Input: dimensioned drawing with shaded views. Units: mm. Origin: part minimum x, y, z. A direction names the side the tool comes from. Give positions to 0.01 mm unless a question says otherwise; leave off trailing zeros. Write each loop counter-clockwise with the first axis right and the second up, starting at its lowest first coordinate (ties: lowest second). Pieces come first, ordered by that corner, then holes. Notation, with made-up numbers: M 25.25,-30 L 34.25,-30 A8 cw 34.25,-16 Z; hole C -34.5,22 d9. An arc over 180 degrees is marked long. Use CSV: the item, a comma, the result in double quotes. Start each with the question number.
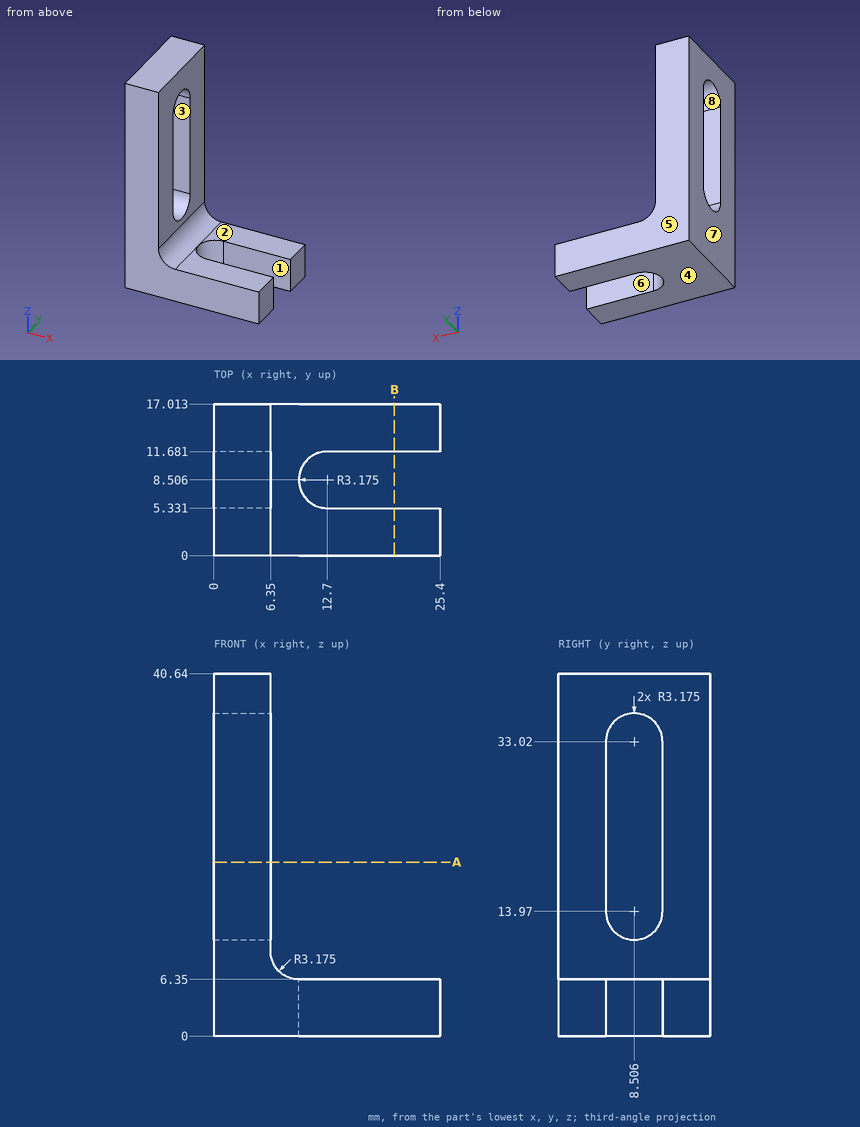
Q1. Section B-B, the plane x = 20.25. Return the cut outline in (y, z).
Q2. Set-up query: the marked faces 1, 2, 3 and 4. Return all of +Z, -Z, +X, -X, +Y, -Y with unobstructed straight access to the full face (end or side cutting, diameter ignored); none if empty.
Q3. Pull-direction query (Y, two-part tool) for the marked faces 5, 6, 7 and 8; classes: released by +Y, released by -Y, zero draft, split by the parting line, or undercut.
Q4. Material intervals for L1, parallel to X at y = 2, z = 32.5; L2, parallel to Z at x = 5.25, y = 7 (1 decimal), sorted ascending. Write a range as [from, to].
Q5. First-contact query: pin 1 Ø5 at (y, z) = (12.5, 36.5) entering from +X; pin 2 Ø4 at (y, z) = (4, 9) entering from +X; pin 3 Ø2.5 at (x, y) = (14.5, 14) entering from +Z. Flat tips, straight axial feed; report the tip coordinate or a pass-through.
Q6. Section A-A, the plane z = 19.5. Return the cut outline in (x, y).
Check result:
1,outline,"M 0,0 L 5.33,0 L 5.33,6.35 L 0,6.35 Z; M 11.68,0 L 17.01,0 L 17.01,6.35 L 11.68,6.35 Z"
2,face 1,"+Z, -Z, +X"
2,face 2,"+Z, +X, +Y, -Y"
2,face 3,"+X, -X"
2,face 4,"-Z, +X, -X, +Y, -Y"
3,face 5,"released by +Y"
3,face 6,"undercut"
3,face 7,"zero draft"
3,face 8,"undercut"
4,L1,"x = [0, 6.35]"
4,L2,"z = [0, 11.2], [35.8, 40.6]"
5,pin 1,"stops at x = 6.35"
5,pin 2,"stops at x = 7.6"
5,pin 3,"stops at z = 6.35"
6,outline,"M 0,0 L 6.35,0 L 6.35,5.33 L 0,5.33 Z; M 0,11.68 L 6.35,11.68 L 6.35,17.01 L 0,17.01 Z"
